Autodesk Inventor part; units mm, degrees
ref_plane "YZ Plane" through (0, 0, 0) normal (1, 0, 0) x (0, 1, 0)
ref_plane "XZ Plane" through (0, 0, 0) normal (0, 1, 0) x (-1, 0, 0)
ref_plane "XY Plane" through (0, 0, 0) normal (0, 0, 1) x (1, 0, 0)
sketch "スケッチ1" plane through (0, 0, 0) normal (1, 0, 0) x (0, 1, 0)
  line L0 (0, 0) -> (5.1, 0)
  line L1 (5.1, 0) -> (5.1, -1.5)
  line L2 (5.1, -1.5) -> (11, -1.5)
  line L3 (11, -1.5) -> (11, -5)
  line L4 (11, -5) -> (5.1, -5)
  line L5 (5.1, -5) -> (5.1, -15)
  line L6 (5.1, -15) -> (4, -15)
  line L7 (4, -15) -> (4, 0)
  line L8 (0, -18) -> (0, 3)
  dimension "d0" = 4
  dimension "d1" = 1.5
  dimension "d2" = 3.5
  dimension "d3" = 10
  dimension "d4" = 11
  dimension "d5" = 5.1
revolve "回転1" add sketch "スケッチ1" angle 360 about axis through (0, 0, -10) along (0, 0, 1)
sketch "スケッチ2" plane through (0, 0, -1.5) normal (0, 0, 1) x (1, 0, 0)
  circle A0 centre (0, 0) radius 8
  point P0 (0, 8)
  point P1 (-8, 0)
  point P2 (0, -8)
  point P3 (8, 0)
  dimension "d7" = 16
  dimension "d10" = 360
hole "穴1" at (0, 8, -1.5) at (-8, 0, -1.5) at (0, -8, -1.5) at (8, 0, -1.5) direction (0, 0, -1) diameter 3.4 end through all
thread "ねじ1"
properties part number "lead-screw-nut" material "真鍮、ソフト イエロー"
The listing builds one solid part. Answer for the finished solid, in the listing's coordinates (mm). A direction names the side the tool comes from. Round coordinates to 2 decimals unless told otherwise and drop trailing zeros. Write each loop counter-clockwise with the first axis right and the second up, starting at its lowest first coordinate (ties: lowest second). Pieces come first, ordered by that corner, then holes. Notation, with made-up numbers: (-25, 44) -> (29, 44) arc R17 cw to (29, 55) -> close; hole circle Ø8 at (-23, -24). An arc over 180 degrees is marked (long way). Answer as a JSON object with one key per item and string values. Group by question number.
Q1. Which of the six approach directions +Z, -Z, +X, -X, +Y, -Y give full straight-line access (tool end or side, diameter ignored) to faces 1 (the face through (-4.5, 2.4, -0.8)), 2 (the face through (-4.5, 2.4, -10.1)), 3 (the face through (3, -3, 0))?
Q2. Section C-C (y = -8) is taken. Write down the section's boundary in (x, z).
Q3. Section A-A (y = 0) is taken. Write down the section's boundary in (x, z), plus the area to 3 significant figures.
Q4. Section B-B (x = 7.5) is taken. Write down the section's boundary in (y, z), plus the area to 3 significant figures.
Q5. Each of these flat-tipped pins is pushed along its axis until it touches: pin 1 Ø5.5 at (x, y) = (-8, 0) entering from +Z; pin 2 Ø1.5 at (x, z) = (8.5, -4) entering from -Y; pin 3 Ø5 at (x, z) = (-1, -5) entering from -Y; pin 4 Ø6 at (x, z) = (-7, -9.5) entering from +Y. Where does it stop, or does it pass through?
Q6. Straight lines are drawn through the part: line 1 along X through (y, z) = (0, -3.9); line 2 along X through (y, z) = (0, -5.25). For each, find the intervals that lie inside material, in ascending order.
Q7. Determine the mould class of faces 4 (the face through (2, 5, -1.5)), 5 (the face through (-10.74, -2.38, -3.27)), 6 (the face through (3.905, -0.867, -7.395)) for opening direction X: pulls with the +X half, pulls with the -X half, needs draft (parallel to the pull), parting line crosses it, or undercut.
Q8. Section D-D (z = -7) is taken. Write down the section's boundary in (x, y), plus the area to 3 significant figures.
Check values:
{
 "1": {"face 1": "+Z", "face 2": "-Z", "face 3": "+Z, +X, -X, +Y, -Y"},
 "2": {"outline": "(-7.55, -5) -> (-1.7, -5) -> (-1.7, -1.5) -> (-7.55, -1.5) -> close; (1.7, -5) -> (7.55, -5) -> (7.55, -1.5) -> (1.7, -1.5) -> close"},
 "3": {"outline": "(-11, -5) -> (-9.7, -5) -> (-9.7, -1.5) -> (-11, -1.5) -> close; (-6.3, -5) -> (-5.1, -5) -> (-5.1, -15) -> (-4, -15) -> (-4, 0) -> (-5.1, 0) -> (-5.1, -1.5) -> (-6.3, -1.5) -> close; (4, -15) -> (5.1, -15) -> (5.1, -5) -> (6.3, -5) -> (6.3, -1.5) -> (5.1, -1.5) -> (5.1, 0) -> (4, 0) -> close; (9.7, -5) -> (11, -5) -> (11, -1.5) -> (9.7, -1.5) -> close", "area": "50.5 mm^2"},
 "4": {"outline": "(-8.05, -5) -> (-1.62, -5) -> (-1.62, -1.5) -> (-8.05, -1.5) -> close; (1.62, -5) -> (8.05, -5) -> (8.05, -1.5) -> (1.62, -1.5) -> close", "area": "45.0 mm^2"},
 "5": {"pin 1": "z = -1.5", "pin 2": "y = -7.81", "pin 3": "y = -11", "pin 4": "y = 3.16"},
 "6": {"line 1": "-11 to -9.7, -6.3 to -4, 4 to 6.3, 9.7 to 11", "line 2": "-5.1 to -4, 4 to 5.1"},
 "7": {"face 4": "needs draft", "face 5": "parting line crosses it", "face 6": "undercut"},
 "8": {"outline": "circle Ø10.2 at (0, 0); hole circle Ø8 at (0, 0)", "area": "31.4 mm^2"}
}
